Can you work these out from the model? Positions are in its coordinate system, mm. Round coordinates to 2 decimals unless told otherwise and drop trailing zeros. Loops run counter-clockwise (first coordinate to the right, second up) from the corner with the lowest first, then second, coordinate; pieces in that order, holes last.
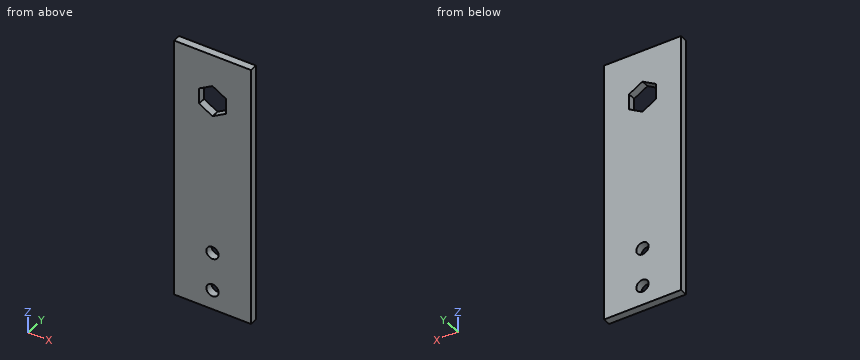
```python
from build123d import *

# Parameters (mm, degrees)
F0_W     = 50
F0_H     = 170
F0_R     = 4
F1_DEPTH = 5


with BuildPart() as f1:
    # F0 (on Front) → F1 (new body)
    with BuildSketch(Plane.XZ):
        with Locations((25, 85)):
            Rectangle(F0_W, F0_H)
        with Locations((25, 12.7)):
            Circle(F0_R, mode=Mode.SUBTRACT)
        with Locations((25, 37.7)):
            Circle(F0_R, mode=Mode.SUBTRACT)
        Polygon((25, 149.381979), (33.73125, 144.34099), (33.73125, 134.25901), (25, 129.218021), (16.26875, 134.25901), (16.26875, 144.34099), align=None, mode=Mode.SUBTRACT)
    extrude(amount=F1_DEPTH)


solid = f1.part
```
(1) Suppose I cut it at A-A (z = 12.7). Write out the boundary of the cut face in (x, y), then the cut area to 3 significant figures.
(2) If I drill on line 1 (Z direction, x = 25, y = -2.55); line 2 (Z direction, x = 24.5, y = -3.1); line 3 (X direction, y = -3.8, z = 137), over which ranges is the centre line in solid material (lowest first)?
(3) For pin 1 (1 mm diameter, centred on x = 27, y = -2, fed in from -Z), with a flat end and sliding along its axis, tell me the tip position at first contact or that it passes through.
(4) Suppose I cut it at B-B (y = -1.45). Write out the boundary of the cut face in (x, z).
Check result:
1. outline: (0, -5) - (21, -5) - (21, 0) - (0, 0) - close; (29, -5) - (50, -5) - (50, 0) - (29, 0) - close
1. area: 210 mm2
2. line 1: z = 0 to 8.7, 16.7 to 33.7, 41.7 to 129.22, 149.38 to 170
2. line 2: z = 0 to 8.73, 16.67 to 33.73, 41.67 to 129.51, 149.09 to 170
2. line 3: x = 0 to 16.27, 33.73 to 50
3. pin 1: stops at z = 0
4. outline: (0, 0) - (50, 0) - (50, 170) - (0, 170) - close; hole (16.27, 134.26) - (25, 129.22) - (33.73, 134.26) - (33.73, 144.34) - (25, 149.38) - (16.27, 144.34) - close; hole circle Ø8 at (25, 12.7); hole circle Ø8 at (25, 37.7)
